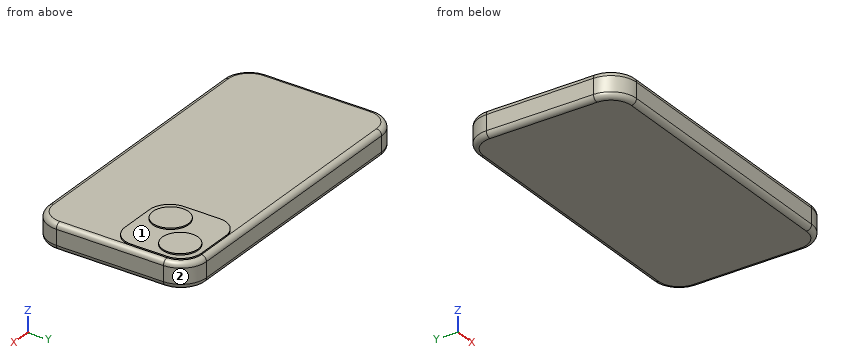
from build123d import *

# Parameters (mm, degrees)
SKETCH1_W           = 152.4
SKETCH1_H           = 78.74
BOSS_EXTRUDE1_DEPTH = 6.35
FILLET1_R           = 12.7
FILLET2_R           = 2.54
BOSS_EXTRUDE2_DEPTH = 0.635
SKETCH3_R           = 8.89
BOSS_EXTRUDE3_DEPTH = 0.635


with BuildPart() as part:
    # Sketch1 → Boss-Extrude1 (new body, symmetric)
    with BuildSketch(Plane.XY):
        Rectangle(SKETCH1_W, SKETCH1_H)
    extrude(amount=BOSS_EXTRUDE1_DEPTH, both=True)

    # Fillet1
    fillet1_edges = [part.edges().sort_by_distance(p)[0] for p in [
        (76.2, -39.37, 0),
        (-76.2, -39.37, 0),
        (-76.2, 39.37, 0),
        (76.2, 39.37, 0),
    ]]
    fillet(fillet1_edges, radius=FILLET1_R)

    # Fillet2
    fillet2_edges = [part.edges().sort_by_distance(p)[0] for p in [
        (0, 39.37, -6.35),
        (0, 39.37, 6.35),
        (76.2, 0, -6.35),
        (0, -39.37, -6.35),
        (-76.2, 0, -6.35),
        (-72.480256121, 35.650256121, -6.35),
        (-72.480256121, -35.650256121, -6.35),
        (72.480256121, -35.650256121, -6.35),
        (72.480256121, 35.650256121, -6.35),
        (76.2, 0, 6.35),
        (-76.2, 0, 6.35),
        (0, -39.37, 6.35),
        (-72.480256121, 35.650256121, 6.35),
        (-72.480256121, -35.650256121, 6.35),
        (72.480256121, -35.650256121, 6.35),
        (72.480256121, 35.650256121, 6.35),
    ]]
    fillet(fillet2_edges, radius=FILLET2_R)

    # Sketch2 → Boss-Extrude2 (add, symmetric)
    with BuildSketch(Plane.XY.offset(6.35)):
        with BuildLine():
            ThreePointArc((73.66, 26.67), (70.684204897, 33.854204897), (63.5, 36.83))
            Line((63.5, 36.83), (45.72, 36.83))
            ThreePointArc((45.72, 36.83), (38.535795103, 33.854204897), (35.56, 26.67))
            Line((35.56, 26.67), (35.56, 8.89))
            ThreePointArc((35.56, 8.89), (38.535795103, 1.705795103), (45.72, -1.27))
            Line((45.72, -1.27), (63.5, -1.27))
            ThreePointArc((63.5, -1.27), (70.684204897, 1.705795103), (73.66, 8.89))
            Line((73.66, 8.89), (73.66, 26.67))
        make_face()
    extrude(amount=BOSS_EXTRUDE2_DEPTH, both=True)

    # Sketch3 → Boss-Extrude3 (add, symmetric)
    with BuildSketch(Plane.XY.offset(6.985)):
        with Locations((62.333473824, 25.503473824)):
            Circle(SKETCH3_R)
        with Locations((47.067038418, 10.237038418)):
            Circle(SKETCH3_R)
    extrude(amount=BOSS_EXTRUDE3_DEPTH, both=True)


solid = part.part
Geometry: final body of the model. Coordinates: model frame, mm. Face numbers are marked on the shaded views. A direction names the side the tool comes from. Give positions to 0.01 mm unless a question says otherwise; leave off trailing zeros. Order: outer loops, then holes, each group sorted by start corner. A loop starts at its lowest first (then second) coordinate and runs counter-clockwise, first axis right, second up. Notation, with made-up numbers: (71.25, 48.25) -> (109.25, 48.25) arc R24 ccw to (109.25, 80.25) -> close; hole circle Ø3 at (44.25, 67). An arc over 180 degrees is marked (long way). Put each result on its own line as item: value.
Q1. Section B-B, the plane y = -16.5. Return loops of the section in (x, z), then the cut area to 3 significant figures.
Here are the results:
outline: (-76.2, -3.81) arc R2.54 ccw to (-73.66, -6.35) -> (73.66, -6.35) arc R2.54 ccw to (76.2, -3.81) -> (76.2, 3.81) arc R2.54 ccw to (73.66, 6.35) -> (-73.66, 6.35) arc R2.54 ccw to (-76.2, 3.81) -> close
area: 1,930 mm^2
Q2. Pin query (flat end, axial travel): pin 1 (5 mm diameter, centred on x = -26.5, y = 24, fed in from +Z); pin 2 (8 mm diameter, centred on y = 20, z = -4.5, fed in from +X); pin 3 (1 mm diameter, centred on y = 30.5, z = 1, fed in from +X). Return the tip coordinate at first contact, or that it passes through.
Here are the results:
pin 1: stops at z = 6.35
pin 2: stops at x = 76.2
pin 3: stops at x = 75.76
Q3. Section C-C, the plane y = 22. Return loops of the section in (x, z) (3 decimals), then the cut area to 3 significant figures.
Here are the results:
outline: (-76.2, -3.81) arc R2.54 ccw to (-73.66, -6.35) -> (73.66, -6.35) arc R2.54 ccw to (76.2, -3.81) -> (76.2, 3.81) arc R2.54 ccw to (73.66, 6.35) -> (73.66, 6.985) -> (70.504, 6.985) -> (70.504, 7.62) -> (54.163, 7.62) -> (54.163, 6.985) -> (35.56, 6.985) -> (35.56, 6.35) -> (-73.66, 6.35) arc R2.54 ccw to (-76.2, 3.81) -> close
area: 1,960 mm^2
Q4. Reachability of the marked faces 1 and 2 from +Z, -Z, +X, -X, +Y, -Y: full face, straight path, thin tool, end or side. Return the list, or none.
Here are the results:
face 1: +Z
face 2: +Z, -Z, +X, +Y
Q5. Section A-A, the plane x = 29.5. Return loops of the section in (y, z), then the cut area to 3 significant figures.
Here are the results:
outline: (-39.37, -3.81) arc R2.54 ccw to (-36.83, -6.35) -> (36.83, -6.35) arc R2.54 ccw to (39.37, -3.81) -> (39.37, 3.81) arc R2.54 ccw to (36.83, 6.35) -> (-36.83, 6.35) arc R2.54 ccw to (-39.37, 3.81) -> close
area: 994 mm^2
Q6. Material intervals for L1, parallel to Z at x = 43.5, y = -14; L2, parallel to X at y = 24.5, z = 6.75; L3, parallel to Y at x = -45, z = -4, sorted ascending.
Here are the results:
L1: z = -6.35 to 6.35
L2: x = 35.56 to 73.66
L3: y = -39.36 to 39.36
